Check sheet for the modelled part. Datum: model origin and axes. Units: mm. Face numbers are marked on the shaded views. A direction names the side the tool comes from. Coordinates: 2 decimals unless noted, no trailing zeros. Write each loop counter-clockwise with the first axis right and the second up, starting at its lowest first coordinate (ties: lowest second). Pieces come first, ordered by that corner, then holes. Notation, with made-up numbers: (-8.5, 39.25) -> (-4.5, 39.25) arc R23 ccw to (-4.5, 55.25) -> close; hole circle Ø8 at (-23.75, 67.25). An arc over 180 degrees is marked (long way). Put each result on its own line as item: value.
Autodesk Inventor part; units mm, degrees
ref_plane "YZ Plane" through (0, 0, 0) normal (1, 0, 0) x (0, 1, 0)
ref_plane "XZ Plane" through (0, 0, 0) normal (0, 1, 0) x (-1, 0, 0)
ref_plane "XY Plane" through (0, 0, 0) normal (0, 0, 1) x (1, 0, 0)
sketch "Sketch1" plane through (0, 0, 0) normal (0, 0, 1) x (1, 0, 0)
  line L0 (0, -5) -> (0, 4.2702)
  line L1 (3.75, -9.2702) -> (3.75, -5)
  line L2 (3.75, -5) -> (0, -5)
  line L3 (3.75, 9.2702) -> (3.75, 4.2702)
  line L4 (3.75, 4.2702) -> (0, 4.2702)
  arc A0 (3.75, -9.2702) -> (3.75, 9.2702) centre (0, 0) ccw
  dimension "d4" = 5
  dimension "d9" = 20
revolve "Revolution1" add sketch "Sketch1" angle 360 about axis through (0, -5, 0) along (0, 1, 0)
sketch "Sketch2" plane through (0, 0, 0) normal (1, 0, 0) x (0, 1, 0)
  circle A0 centre (0, 0) radius 3.75
  dimension "d11" = 7.5
extrude "Extrusion1" cut sketch "Sketch2" along normal blind 10
sketch "Sketch3" plane through (0, 0, 0) normal (1, 0, 0) x (0, 0, -1)
  circle A0 centre (0, 0) radius 3.75
extrude "Extrusion2" add sketch "Sketch3" along normal blind 4.27
sketch "Sketch4" plane through (0, 0, 0) normal (0, 0, 1) x (1, 0, 0)
  circle A0 centre (0, 0) radius 3.75
  dimension "d16" = 7.5
extrude "Extrusion3" cut sketch "Sketch4" along normal blind 10
sketch "Sketch5" plane through (0, 0, 0) normal (0, 0, 1) x (1, 0, 0)
  circle A0 centre (0, 0) radius 3.75
extrude "Extrusion4" add sketch "Sketch5" along normal blind 4.27
properties part number "Base2"
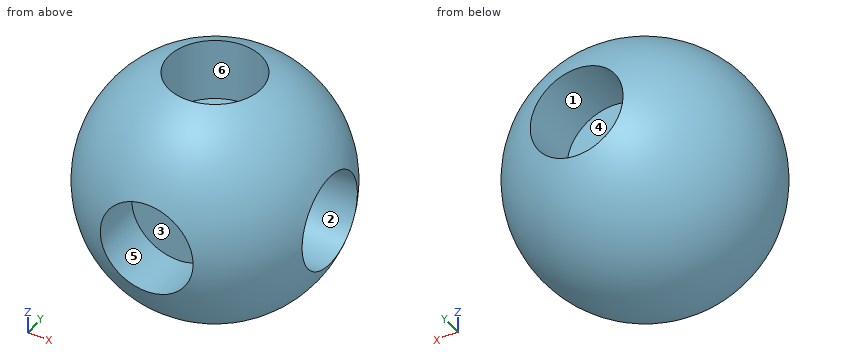
Q1. Tool access check on the marked faces 4, 5 and 6. Record the directions out of +Z, -Z, +X, -X, +Y, -Y that give a thin tool (end or side, any length) a straight path to the whole face; none if there is none.
Recorded:
face 4: +Y
face 5: -Y
face 6: +Z
Q2. Cross-section at B-B (x = 0). Record the cut outline in (y, z), plus the area to 3 significant figures.
Recorded:
outline: (-9.27, -3.75) arc R10 ccw to (9.27, -3.75) -> (4.27, -3.75) -> (4.27, 3.75) -> (9.27, 3.75) arc R10 ccw to (3.75, 9.27) -> (3.75, 4.27) -> (-3.75, 4.27) -> (-3.75, 9.27) arc R10 ccw to (-9.27, 3.75) -> (-5, 3.75) -> (-5, -3.75) -> close
area: 196 mm2
Q3. Cross-section at A-A (y = 0). Record the cut outline in (x, z).
Recorded:
outline: (-3.75, 4.27) -> (-3.75, 9.27) arc R10 ccw (long way) to (9.27, -3.75) -> (4.27, -3.75) -> (4.27, 3.75) -> (9.27, 3.75) arc R10 ccw to (3.75, 9.27) -> (3.75, 4.27) -> close
Q4. Material ranges on line 1 along Y through (x, z) = (2.5, 2.5); line 2 along Z through (x, y) = (0, 5.8); line 3 along X through (y, z) = (6.5, 0), recorded low to high.
Recorded:
line 1: y = -5 to 4.27
line 2: z = -8.15 to -3.75, 3.75 to 8.15
line 3: x = -7.6 to -3.75, 3.75 to 7.6
Q5. Cross-section at C-C (z = 0). Record the cut outline in (x, y).
Recorded:
outline: (-3.75, -9.27) -> (-3.75, -5) -> (3.75, -5) -> (3.75, -9.27) arc R10 ccw to (9.27, -3.75) -> (4.27, -3.75) -> (4.27, 3.75) -> (9.27, 3.75) arc R10 ccw to (3.75, 9.27) -> (3.75, 4.27) -> (-3.75, 4.27) -> (-3.75, 9.27) arc R10 ccw to start
Q6. Mould release check, pull along Y, two halves, no side actions. Record for the marked faces 1, 2 and 3: released by +Y, released by -Y, zero draft, split by the parting line, or undercut.
Recorded:
face 1: zero draft
face 2: undercut
face 3: released by -Y
Q7. Depth check by flat-ended pin: P1, Ø4, axis at x = -5, y = 3.5, coming from the +Z side; P2, Ø4, axis at y = 0, z = -2.5, coming from the -X side; P3, Ø6, axis at x = 0, z = 0, coming from the +Y side. Enter the tip coordinate at first touch or a pass-through.
Recorded:
P1: stops at z = 9.12
P2: stops at x = -9.99
P3: stops at y = 4.27
Q8. Cross-section at D-D (x = 6.25). Record the cut outline in (y, z).
Recorded:
outline: circle Ø15.61 at (0, 0); hole circle Ø7.5 at (0, 0)
